Read the model definition and answer for the solid it produces. Units are mm, in the model's axes. A direction names the side the tool comes from. Give positions to 0.01 mm unless a question says otherwise; leave off trailing zeros. Write each loop counter-clockwise with the first axis right and the second up, starting at its lowest first coordinate (ties: lowest second). Pieces come first, ordered by that corner, then holes. Notation, with made-up numbers: (24.5, 41) -> (39.5, 41) arc R14 cw to (39.5, 64) -> close; hole circle Ø10 at (-38.75, 5). An arc over 180 degrees is marked (long way). Write item = value, one per line.
from build123d import *

# Parameters (mm, degrees)
EXTRUDE_THIN1_DEPTH                       = 9.525
SKETCH4_R                                 = 3.175
CUT_EXTRUDE1_DEPTH                        = 61.325
CSK_FOR_8_FLAT_HEAD_MACHINE_SCREW_2_COUNT = 2
CSK_FOR_8_FLAT_HEAD_MACHINE_SCREW_2_PITCH = 17.4625
CSK_FOR_8_FLAT_HEAD_MACHINE_SCREW_3_COUNT = 2
CSK_FOR_8_FLAT_HEAD_MACHINE_SCREW_3_PITCH = 34.925
FILLET1_R                                 = 6.35


with BuildPart() as part:
    # Sketch2 → Extrude-Thin1 (new body, symmetric)
    with BuildSketch(Plane(origin=(0, 0, 66.675), x_dir=(0, -1, 0), z_dir=(1, 0, 0))):
        with BuildLine():
            Line((22.225, 66.675), (-22.225, 66.675))
            ThreePointArc((-22.225, 66.675), (-32.15743925, 61.88933197), (-34.604310473, 51.139039455))
            Line((-34.604310473, 51.139039455), (-25.720689527, 12.360960545))
            ThreePointArc((-25.720689527, 12.360960545), (-25.480427048, 10.952017343), (-25.4, 9.525))
            Line((-25.4, 9.525), (-25.4, -9.525))
            Line((-25.4, -9.525), (-22.225, -9.525))
            Line((-22.225, -9.525), (-22.225, 9.525))
            ThreePointArc((-22.225, 9.525), (-22.325533809, 11.308771679), (-22.625861909, 13.069950682))
            Line((-22.625861909, 13.069950682), (-31.509482855, 51.848029591))
            ThreePointArc((-31.509482855, 51.848029591), (-29.674329438, 59.910748978), (-22.225, 63.5))
            Line((-22.225, 63.5), (22.225, 63.5))
            Line((22.225, 63.5), (22.225, 66.675))
        make_face()
    extrude_thin1 = extrude(amount=EXTRUDE_THIN1_DEPTH, both=True)

    # Mirror1: Extrude-Thin1 across plane
    add(extrude_thin1.mirror(Plane.ZX))

    # Sketch4 → Cut-Extrude1 (cut, through all)
    with BuildSketch(Plane.XZ.offset(25.4)):
        with Locations((0, 66.675)):
            Circle(SKETCH4_R)
    extrude(amount=-CUT_EXTRUDE1_DEPTH, mode=Mode.SUBTRACT)

    # Sketch6 → CSK for #8 Flat Head Machine Screw (100)1 (revolve, cut)
    with BuildSketch(Plane(origin=(0, -17.4625, 3.175), x_dir=(0, -1, 0), z_dir=(1, 0, 0))):
        Polygon((0, 0), (0, 3.175), (2.45745, 3.175), (2.45745, 1.475934296), (4.2164, 0), align=None)
    csk_for_8_flat_head_machine_screw_100 = revolve(axis=Axis((0, -17.4625, 9.525), (0, 0, -1)), mode=Mode.SUBTRACT)

    # CSK for _8 Flat Head Machine Screw _ 2: CSK for #8 Flat Head Machine Screw (100)1 ×2
    with Locations(*[(0, i * CSK_FOR_8_FLAT_HEAD_MACHINE_SCREW_2_PITCH, 0) for i in range(1, CSK_FOR_8_FLAT_HEAD_MACHINE_SCREW_2_COUNT)]):
        add(csk_for_8_flat_head_machine_screw_100, mode=Mode.SUBTRACT)

    # CSK for _8 Flat Head Machine Screw _ 3: CSK for #8 Flat Head Machine Screw (100)1 ×2
    with Locations(*[(0, i * CSK_FOR_8_FLAT_HEAD_MACHINE_SCREW_3_PITCH, 0) for i in range(1, CSK_FOR_8_FLAT_HEAD_MACHINE_SCREW_3_COUNT)]):
        add(csk_for_8_flat_head_machine_screw_100, mode=Mode.SUBTRACT)

    # Fillet1
    fillet1_edges = [part.edges().sort_by_distance(p)[0] for p in [
        (-9.525, 23.8125, 76.2),
        (9.525, -23.8125, 76.2),
        (-9.525, -23.8125, 76.2),
        (9.525, 23.8125, 76.2),
    ]]
    fillet(fillet1_edges, radius=FILLET1_R)


solid = part.part
(1) The part is cut by section A-A on y = 0. Determine the outline of the cut face in (x, z) (3 decimals).
Checks:
outline = (-9.525, 0) -> (-2.457, 0) -> (-2.457, 1.699) -> (-4.216, 3.175) -> (-9.525, 3.175) -> close; (2.457, 0) -> (9.525, 0) -> (9.525, 3.175) -> (4.216, 3.175) -> (2.457, 1.699) -> close
(2) Given P1, Ø3, axis at x = 0, y = 17.46, coming from the +Z side; P2, Ø6, axis at x = 6, z = 62, coming from the -Y side; P3, Ø3, axis at x = 0.5, z = 68.5, coming from the +Y side; P4, Ø5.5, axis at x = -2, y = -3.5, coming from the +Z side (3 decimals), each flat-ended and moving along its own axis, determine where each tip first touches the part or whether it passes through.
Checks:
P1 = through
P2 = -25.4
P3 = 25.4
P4 = 3.175
(3) The part is cut by section D-D on z = 65. Determine the outline of the cut face in (x, y) (3 decimals), plus the area to 3 significant figures.
Checks:
outline = (-9.525, -25.4) -> (-2.697, -25.4) -> (-2.697, -22.225) -> (-9.525, -22.225) -> close; (-9.525, 22.225) -> (-2.697, 22.225) -> (-2.697, 25.4) -> (-9.525, 25.4) -> close; (2.697, -25.4) -> (9.525, -25.4) -> (9.525, -22.225) -> (2.697, -22.225) -> close; (2.697, 22.225) -> (9.525, 22.225) -> (9.525, 25.4) -> (2.697, 25.4) -> close
area = 86.7 mm²
(4) The part is cut by section C-C on x = 0. Count the separate pieces of the cut face and the enclosed holes in it, plus the area to 3 significant figures.
Checks:
separate_pieces = 6
enclosed_holes = 0
area = 567 mm²
(5) The part is cut by section B-B on z = 28. Determine the outline of the cut face in (x, y) (3 decimals).
Checks:
outline = (-9.525, -31.749) -> (9.525, -31.749) -> (9.525, -28.492) -> (-9.525, -28.492) -> close; (-9.525, 28.492) -> (9.525, 28.492) -> (9.525, 31.749) -> (-9.525, 31.749) -> close
(6) Consider L1, parallel to Y at x = -6.5, z = 59.5 (3 decimals); L2, parallel to Z at x = 8, y = -10 (3 decimals); L3, parallel to Y at x = -6, z = 18.5. Determine where each line is inside the solid, lowest interval first.
Checks:
L1 = -25.4 to -22.225, 22.225 to 25.4
L2 = 0 to 3.175
L3 = -33.93 to -30.67, 30.67 to 33.93
(7) A tool of negligible diameter and unlimited length cuts with its end or side. For faces 1 (the flat face through (0.133, -27.005, 34.487)), 2 (the flat face through (4, 0, 0)), 3 (the flat face through (4.4, 0.3, 3.175)), 4 (the flat face through (2, 25.4, 64)), from which of +Z, -Z, +X, -X, +Y, -Y can it reach the whole face along a straight path? Write none if from no direction.
Checks:
face_1 = +X, -X
face_2 = -Z, +X, -X, +Y, -Y
face_3 = +Z, +X, -X
face_4 = +Z, +X, -X, +Y
(8) For a pull along X with two mould halves and no side action, classify faces 5 (the cylindrical face through (-0.108, 19.918, 0.861)), 6 (the cylindrical face through (-0.688, -23.835, 63.576)), 7 (the cylindrical face through (0.133, -32.057, 4.661)), 8 (the cylindrical face through (-7.714, -23.79, 74.29)) as released by +X, released by -X, zero draft, split by the parting line, or undercut.
Checks:
face_5 = undercut
face_6 = undercut
face_7 = zero draft
face_8 = released by -X
